For this review, take the finished solid that the model builds, in its own axes (mm). A direction names the side the tool comes from. Coordinates: 2 decimals unless noted, no trailing zeros. Loops run counter-clockwise (first coordinate to the right, second up) from the corner with the lowest first, then second, coordinate; pieces in that order, holes last. Notation, with made-up numbers: (-0.5, -18.75) - (16.5, -18.75) arc R23 cw to (16.5, -2.75) - close; hole circle Ø1 at (-19, 36). An arc over 180 degrees is marked (long way). Use one line per item in the form item = value. Start each with the question number.
1. Machinability: for faces 1 (the face through (-42, 42, 15)), 2 (the face through (41, 42, 15)), 3 (the face through (14, 41, 1)), which of the approach directions +Z, -Z, +X, -X, +Y, -Y give a long, thin tool a straight path to every point of the face, cutting with its end or side? Answer none if there is none.
2. For pin 1 Ø19.5 at (x, y) = (-0.5, 52.5) entering from -Z; pin 2 Ø12 at (x, y) = (-49.98, 66) entering from +Z; pin 3 Ø17 at (x, y) = (50.02, 16) entering from +Z, all flat-tipped, find the tip position at first contact; note any pin that passes through.
3. Add section D-D on y = 46. Give the boundary of the cut face in (x, z).
4. Draft analysis for pull direction Y (two halves, no side actions). For faces 4 (the face through (14, 41, 16)), 5 (the face through (-44.452, 60.931, 7.605)), 6 (the face through (66.48, 1.43, 7.6)), state which applies: +Y half, -Y half, draft (parallel to the pull), parting line (faces both ways), or undercut.
5. Add section A-A on y = 66. Give the boundary of the cut face in (x, z), and give its area (3 significant figures).
6. Add section B-B on x = 50.02. Give the boundary of the cut face in (y, z), and give its area (3 significant figures).
7. Add section C-C on z = 7. Give the boundary of the cut face in (x, y).
8. To check wall thickness, follow probe 1 along Y at (x, z) = (50.02, 5.5); probe 2 along X at (y, z) = (66, 5.75); probe 3 along Y at (x, z) = (-49, 13). State the ranges of each line that lie inside material, in increasing order.
```python
from build123d import *

# Parameters (mm, degrees)
F1_DEPTH = 15
F4_DEPTH = 83.051
F7_DEPTH = 83.05
F8_R     = 5
F10_D    = 15


with BuildPart() as f1:
    # F0 (on Top) → F1 (new body)
    with BuildSketch(Plane.XY):
        Polygon((-67.98, 0), (0, 0), (67.98, 0), (67.98, 83.05), (-67.98, 83.05), align=None)
    extrude(amount=F1_DEPTH)

    # F3 (on offset) → F4 (cut, through all)
    with BuildSketch(Plane.XZ):
        Polygon((-15, 0), (0, 0), (15, 0), (12.24, 2.76), (-12.24, 2.76), align=None)
    extrude(amount=-F4_DEPTH, mode=Mode.SUBTRACT)

    # F6 (on offset) → F7 (join)
    with BuildSketch(Plane.XZ):
        Polygon((-15, 15), (0, 15), (15, 15), (12.24, 17.76), (-12.24, 17.76), align=None)
    extrude(amount=-F7_DEPTH)

    # F8
    f8_edges = [f1.edges().sort_by_distance(p)[0] for p in [
        (-67.98, 0, 7.5),
        (67.98, 0, 7.5),
        (67.98, 83.05, 7.5),
        (-67.98, 83.05, 7.5),
    ]]
    fillet(f8_edges, radius=F8_R)

    # F10 (through all)
    with Locations(Plane(origin=(0, 0, 0), x_dir=(1, 0, 0), z_dir=(0, 0, -1))):
        with Locations((-49.98, -66), (-49.98, -16), (50.02, -66), (50.02, -16)):
            Hole(F10_D / 2)


solid = f1.part
```
Conclusion:
q1.face_1 = +Z, -X, +Y, -Y
q1.face_2 = +Z, +X, +Y, -Y
q1.face_3 = -Z, +Y, -Y
q2.pin_1 = 2.76
q2.pin_2 = through
q2.pin_3 = 15
q3.outline = (-67.98, 0) - (-15, 0) - (-12.24, 2.76) - (12.24, 2.76) - (15, 0) - (67.98, 0) - (67.98, 15) - (15, 15) - (12.24, 17.76) - (-12.24, 17.76) - (-15, 15) - (-67.98, 15) - close
q4.face_4 = draft
q4.face_5 = undercut
q4.face_6 = -Y half
q5.outline = (-67.98, 0) - (-57.48, 0) - (-57.48, 15) - (-67.98, 15) - close; (-42.48, 0) - (-15, 0) - (-12.24, 2.76) - (12.24, 2.76) - (15, 0) - (42.52, 0) - (42.52, 15) - (15, 15) - (12.24, 17.76) - (-12.24, 17.76) - (-15, 15) - (-42.48, 15) - close; (57.52, 0) - (67.98, 0) - (67.98, 15) - (57.52, 15) - close
q5.area = 1,590 mm^2
q6.outline = (0, 0) - (8.5, 0) - (8.5, 15) - (0, 15) - close; (23.5, 0) - (58.5, 0) - (58.5, 15) - (23.5, 15) - close; (73.5, 0) - (83.05, 0) - (83.05, 15) - (73.5, 15) - close
q6.area = 796 mm^2
q7.outline = (-67.98, 5) arc R5 ccw to (-62.98, 0) - (62.98, 0) arc R5 ccw to (67.98, 5) - (67.98, 78.05) arc R5 ccw to (62.98, 83.05) - (-62.98, 83.05) arc R5 ccw to (-67.98, 78.05) - close; hole circle Ø15 at (-49.98, 16); hole circle Ø15 at (-49.98, 66); hole circle Ø15 at (50.02, 16); hole circle Ø15 at (50.02, 66)
q8.probe_1 = 0 to 8.5, 23.5 to 58.5, 73.5 to 83.05
q8.probe_2 = -67.98 to -57.48, -42.48 to 42.52, 57.52 to 67.98
q8.probe_3 = 0 to 8.56, 23.44 to 58.56, 73.44 to 83.05
